Here's how the part is built. I have some questions about the finished solid (model axes, mm). A direction names the side the tool comes from. Round coordinates to 2 decimals unless told otherwise and drop trailing zeros. Order: outer loops, then holes, each group sorted by start corner. A loop starts at its lowest first (then second) coordinate and runs counter-clockwise, first axis right, second up. Notation, with made-up numbers: (64.25, 44) -> (70.25, 44) arc R17 ccw to (70.25, 48) -> close; hole circle Ø4 at (20.25, 83). An arc over 180 degrees is marked (long way). One line per item, written item: value.
```python
from build123d import *

# Parameters (mm, degrees)
F1_DEPTH = 5
F2_DEPTH = 2
F3_DEPTH = 2
F4_R     = 1
F5_D     = 2


with BuildPart() as f1:
    # F0 (on Top) → F1 (new body)
    with BuildSketch(Plane.XY):
        with BuildLine():
            ThreePointArc((4.582575695, -2), (4.8945315647, -1.0215482184), (5, 0))
            ThreePointArc((5, 0), (-4.8945315647, 1.0215482184), (4.582575695, -2))
        make_face()
    extrude(amount=-F1_DEPTH)

    # F0 (on Top) → F2 (join)
    with BuildSketch(Plane.XY):
        with BuildLine():
            Line((13, 0), (5, 0))
            ThreePointArc((5, 0), (4.8945315647, -1.0215482184), (4.582575695, -2))
            Line((4.582575695, -2), (10.6197060227, -2))
            Line((10.6197060227, -2), (10.6197060227, -4.87568))
            Line((10.6197060227, -4.87568), (15.2, -0.999998501))
            Line((15.2, -0.999998501), (15.2, 0))
            Line((15.2, 0), (13, 0))
        make_face()
    extrude(amount=-F2_DEPTH)

    # F0 (on Top) → F3 (join, symmetric)
    with BuildSketch(Plane.XY):
        with BuildLine():
            Line((13, 0), (5, 0))
            ThreePointArc((5, 0), (4.8945315647, -1.0215482184), (4.582575695, -2))
            Line((4.582575695, -2), (10.6197060227, -2))
            Line((10.6197060227, -2), (10.6197060227, -4.87568))
            Line((10.6197060227, -4.87568), (15.2, -0.999998501))
            Line((15.2, -0.999998501), (15.2, 0))
            Line((15.2, 0), (13, 0))
        make_face()
    extrude(amount=F3_DEPTH, both=True)

    # F4
    f4_edges = [f1.edges().sort_by_distance(p)[0] for p in [
        (10.619706, -4.87568, 0),
        (15.2, -0.999999, 0),
    ]]
    fillet(f4_edges, radius=F4_R)

    # F5 (through all)
    with Locations(Plane.XY):
        with Locations((0, 0)):
            Hole(F5_D / 2)


solid = f1.part
```
Q1. I want a section at B-B on z = 0.5. Write out the boundary of the cut face in (x, y).
Answers:
outline: (4.58, -2) -> (10.62, -2) -> (10.62, -2.72) arc R1 ccw to (12.27, -3.48) -> (14.85, -1.3) arc R1 ccw to (15.2, -0.54) -> (15.2, 0) -> (5, 0) arc R5 cw to start
Q2. For P1, Ø1, axis at x = -1, y = -4, coming from the +Z side; P2, Ø0.8, axis at y = -2.5, z = -1, coming from the -X side; P3, Ø2, axis at x = 9, z = 1, coming from the +Y side, each with a flat end and sliding along its axis, tell me the tip position at first contact or that it passes through.
Answers:
P1: z = 0
P2: x = -4.54
P3: y = 0
Q3. If we mould it in two halves opening along X, with no side actions, what happens to faces 1 (the face through (13.538, -2.407, 0.028)), 2 (the face through (11.21, -3.63, 0.03)), 3 (the face through (10, 0, 0))? For each: pulls with the +X half, pulls with the -X half, needs draft (parallel to the pull), parting line crosses it, or undercut.
Answers:
face 1: pulls with the +X half
face 2: undercut
face 3: needs draft
Q4. I need wall thicknesses on line 1 along Y through (x, z) = (0, -2.35); line 2 along Y through (x, z) = (5.25, -0.5); line 3 along Z through (x, y) = (-4, 2.5). Which ranges of each line are inside material? Lowest first, please.
Answers:
line 1: -5 to -1, 1 to 5
line 2: -2 to 0
line 3: -5 to 0
Q5. Which directions (+Z, -Z, +X, -X, +Y, -Y) give clear straight access to the entire face, cutting with the end or side of a thin tool? Please do faces 4 (the face through (4.9, -1, 1)), 5 (the face through (10, -1, 2)), 6 (the face through (8, -2, 0)).
Answers:
face 4: +Z, -X, +Y
face 5: +Z, +X, -X, +Y, -Y
face 6: +Z, -Z, -Y
Q6. I want a section at D-D on x = 7.75. Write out the boundary of the cut face in (y, z).
Answers:
outline: (-2, -2) -> (0, -2) -> (0, 2) -> (-2, 2) -> close
Q7. I want a section at A-A on x = 0. Write out the boundary of the cut face in (y, z).
Answers:
outline: (-5, -5) -> (-1, -5) -> (-1, 0) -> (-5, 0) -> close; (1, -5) -> (5, -5) -> (5, 0) -> (1, 0) -> close
Q8. I want a section at C-C on y = -1.75. Write out the boundary of the cut face in (x, z).
Answers:
outline: (-4.68, -5) -> (4.68, -5) -> (4.68, -2) -> (14.31, -2) -> (14.31, 2) -> (4.68, 2) -> (4.68, 0) -> (-4.68, 0) -> close
